Geometry check sheet. Reference: the model listing, model coordinates, mm. Coordinates: 2 decimals unless noted, no trailing zeros. Write each loop counter-clockwise with the first axis right and the second up, starting at its lowest first coordinate (ties: lowest second). Pieces come first, ordered by that corner, then holes.
from build123d import *

# Parameters (mm, degrees)
SKETCH1_W           = 110
SKETCH1_H           = 110
BOSS_EXTRUDE1_DEPTH = 5
SKETCH2_W           = 101.5
SKETCH2_H           = 101.5
CUT_EXTRUDE1_DEPTH  = 2
CUT_EXTRUDE2_DEPTH  = 1.1


with BuildPart() as part:
    # Sketch1 → Boss-Extrude1 (new body)
    with BuildSketch(Plane(origin=(0, 0, 0), x_dir=(1, 0, 0), z_dir=(0, 1, 0))):
        with Locations((-13.863013699, -16.650684932)):
            Rectangle(SKETCH1_W, SKETCH1_H)
    extrude(amount=BOSS_EXTRUDE1_DEPTH)

    # Sketch2 → Cut-Extrude1 (cut)
    with BuildSketch(Plane(origin=(0, 5, 0), x_dir=(1, 0, 0), z_dir=(0, 1, 0))):
        with Locations((-13.863013699, -16.650684932)):
            Rectangle(SKETCH2_W, SKETCH2_H)
    extrude(amount=-CUT_EXTRUDE1_DEPTH, mode=Mode.SUBTRACT)

    # Sketch3 → Cut-Extrude2 (cut)
    with BuildSketch(Plane(origin=(0, 3, 0), x_dir=(1, 0, 0), z_dir=(0, 1, 0))):
        Polygon((-34.363013699, 1.849315068), (-36.863013699, 1.849315068), (-36.863013699, 19.449315068), (-52.363013699, 19.449315068), (-52.363013699, 1.849315068), (-54.863013699, 1.849315068), (-54.863013699, -13.650684932), (-52.363013699, -13.650684932), (-52.363013699, -31.250684932), (-36.863013699, -31.250684932), (-36.863013699, -13.650684932), (-34.363013699, -13.650684932), align=None)
    extrude(amount=-CUT_EXTRUDE2_DEPTH, mode=Mode.SUBTRACT)


solid = part.part
1. Sectioned sample at B-B, the plane x = -22. Record the boundary of the cut face in (y, z).
Computed values:
outline: (0, -38.35) - (5, -38.35) - (5, -34.1) - (3, -34.1) - (3, 67.4) - (5, 67.4) - (5, 71.65) - (0, 71.65) - close
2. Draft check along X on faces 1 (the flat face through (-68.863, 2, 17)), 2 (the flat face through (-15, 2, 71.651)), 3 (the flat face through (-15, 3, 16)), 4 (the flat face through (41.137, 2, 17)). Enter one of: released by +X, released by -X, zero draft, split by the parting line, or undercut.
Computed values:
face 1: released by -X
face 2: zero draft
face 3: undercut
face 4: released by +X
3. Sectioned sample at D-D, the plane z = 63.5. Record the boundary of the cut face in (x, y).
Computed values:
outline: (-68.86, 0) - (41.14, 0) - (41.14, 5) - (36.89, 5) - (36.89, 3) - (-64.61, 3) - (-64.61, 5) - (-68.86, 5) - close
4. Gauge pin test, flat end, axial feed: pin 1 Ø10 at (x, z) = (-40.5, 14) entering from +Y. Record the tip position at first contact, or that the pin passes through.
Computed values:
pin 1: stops at y = 3
5. Thickness scan on line 1 along X through (y, z) = (3.4, 48.5); line 2 along Z through (x, y) = (-64, 4.6); line 3 along Z through (x, y) = (-51, 2.85). Record the ranges inside material, lowest first.
Computed values:
line 1: x = -68.86 to -64.61, 36.89 to 41.14
line 2: z = -38.35 to -34.1, 67.4 to 71.65
line 3: z = -38.35 to -19.45, 31.25 to 71.65
6. Sectioned sample at A-A, the plane y = 4. Record the boundary of the cut face in (x, z), and give its area (3 significant figures).
Computed values:
outline: (-68.86, -38.35) - (41.14, -38.35) - (41.14, 71.65) - (-68.86, 71.65) - close; hole (-64.61, -34.1) - (36.89, -34.1) - (36.89, 67.4) - (-64.61, 67.4) - close
area: 1,800 mm2
7. Sectioned sample at C-C, the plane z = 2. Record the boundary of the cut face in (x, y), and give its area (3 significant figures).
Computed values:
outline: (-68.86, 0) - (41.14, 0) - (41.14, 5) - (36.89, 5) - (36.89, 3) - (-34.36, 3) - (-34.36, 1.9) - (-54.86, 1.9) - (-54.86, 3) - (-64.61, 3) - (-64.61, 5) - (-68.86, 5) - close
area: 324 mm2
